from build123d import *

# Parameters (mm, degrees)
CROQUIS1_W              = 35
CROQUIS1_H              = 15
CROQUIS1_R              = 1.5
SALIENTE_EXTRUIR1_DEPTH = 4
CROQUIS2_W              = 4
CROQUIS2_H              = 15
SALIENTE_EXTRUIR2_DEPTH = 60
SALIENTE_EXTRUIR3_DEPTH = 15
CROQUIS4_R              = 2.85
CORTAR_EXTRUIR1_DEPTH   = 1.65
CROQUIS5_W              = 5
CROQUIS5_H              = 22
CORTAR_EXTRUIR2_DEPTH   = 22
CORTAR_EXTRUIR5_REACH   = 73.507
CROQUIS6_R              = 1.5
CROQUIS7_R              = 2.5
CORTAR_EXTRUIR6_DEPTH   = 2
CROQUIS9_W              = 13
CROQUIS9_H              = 14.4
SALIENTE_EXTRUIR4_DEPTH = 10


with BuildPart() as part:
    # Croquis1 → Saliente-Extruir1 (new body)
    with BuildSketch(Plane(origin=(0, 0, 0), x_dir=(1, 0, 0), z_dir=(0, 1, 0))):
        Rectangle(CROQUIS1_W, CROQUIS1_H)
        with Locations(Location((5.5, 3.75, 0), (0, 0, 270))):
            Circle(CROQUIS1_R, mode=Mode.SUBTRACT)
        with Locations(Location((13.5, 3.75, 0), (0, 0, 270))):
            Circle(CROQUIS1_R, mode=Mode.SUBTRACT)
    extrude(amount=SALIENTE_EXTRUIR1_DEPTH)

    # Croquis2 → Saliente-Extruir2 (add)
    with BuildSketch(Plane(origin=(0, 4, 0), x_dir=(1, 0, 0), z_dir=(0, 1, 0))):
        with Locations((-15.5, 0)):
            Rectangle(CROQUIS2_W, CROQUIS2_H)
    extrude(amount=SALIENTE_EXTRUIR2_DEPTH)

    # Croquis3 → Saliente-Extruir3 (add)
    with BuildSketch(Plane.XY.offset(7.5)):
        Polygon((-13.5, 4), (-13.5, 30), (1.5, 4), align=None)
    extrude(amount=-SALIENTE_EXTRUIR3_DEPTH)

    # Croquis4 → Cortar-Extruir1 (cut)
    with BuildSketch(Plane(origin=(0, 4, 0), x_dir=(1, 0, 0), z_dir=(0, 1, 0))):
        with Locations(Location((5.5, 3.75, 0), (0, 0, 270))):
            Circle(CROQUIS4_R)
        with Locations(Location((13.5, 3.75, 0), (0, 0, 270))):
            Circle(CROQUIS4_R)
    extrude(amount=-CORTAR_EXTRUIR1_DEPTH, mode=Mode.SUBTRACT)

    # Croquis5 → Cortar-Extruir2 (cut)
    with BuildSketch(Plane(origin=(17.5, 0, 0), x_dir=(0, 0, -1), z_dir=(1, 0, 0))):
        with Locations((-5, 11)):
            Rectangle(CROQUIS5_W, CROQUIS5_H)
    extrude(amount=-CORTAR_EXTRUIR2_DEPTH, mode=Mode.SUBTRACT)

    # Croquis6 → Cortar-Extruir5 (cut, up to next)
    with BuildSketch(Plane(origin=(-13.5, 0, 0), x_dir=(0, 0, -1), z_dir=(1, 0, 0)), mode=Mode.PRIVATE) as cortar_extruir5_sk1:
        with Locations((-3.3, 59.52)):
            Circle(CROQUIS6_R)
    cortar_extruir5_tool1 = extrude(cortar_extruir5_sk1.sketch, amount=-CORTAR_EXTRUIR5_REACH, mode=Mode.PRIVATE) & part.part
    # Croquis6 → Cortar-Extruir5 (cut, up to next)
    with BuildSketch(Plane(origin=(-13.5, 0, 0), x_dir=(0, 0, -1), z_dir=(1, 0, 0)), mode=Mode.PRIVATE) as cortar_extruir5_sk2:
        with Locations((3.3, 52.48)):
            Circle(CROQUIS6_R)
    cortar_extruir5_tool2 = extrude(cortar_extruir5_sk2.sketch, amount=-CORTAR_EXTRUIR5_REACH, mode=Mode.PRIVATE) & part.part
    add(cortar_extruir5_tool1.solids().sort_by_distance((-13.5, 59.52, 3.3))[0], mode=Mode.SUBTRACT)
    add(cortar_extruir5_tool2.solids().sort_by_distance((-13.5, 52.48, -3.3))[0], mode=Mode.SUBTRACT)

    # Croquis7 → Cortar-Extruir6 (cut)
    with BuildSketch(Plane.ZY.offset(17.5)):
        with Locations((-3.3, 52.48)):
            Circle(CROQUIS7_R)
        with Locations((3.3, 59.52)):
            Circle(CROQUIS7_R)
    extrude(amount=-CORTAR_EXTRUIR6_DEPTH, mode=Mode.SUBTRACT)

    # Croquis9 → Saliente-Extruir4 (add)
    with BuildSketch(Plane.XY.offset(7.5)):
        with Locations((-11, 7.2)):
            Rectangle(CROQUIS9_W, CROQUIS9_H)
    extrude(amount=SALIENTE_EXTRUIR4_DEPTH)


solid = part.part
Input: part model. Units: mm. Frame: model coordinates. A direction names the side the tool comes from. Give positions to 0.01 mm unless a question says otherwise; leave off trailing zeros. Write each loop counter-clockwise with the first axis right and the second up, starting at its lowest first coordinate (ties: lowest second). Pieces come first, ordered by that corner, then holes.
Q1. First-contact query: P1, Ø1, axis at y = 57.5, z = -1, coming from the +X side; P2, Ø3, axis at x = 8.5, z = -1.5, coming from the +Y side; P3, Ø11, axis at x = -14, z = 13.5, coming from the +Y side. Flat tips, straight axial feed; report the tip coordinate or a pass-through.
Q2. Set-up query: faces 4 (the face through (9, 4, -3)), 5 (the face through (-15.5, 51, -2)), 6 (the face through (4, 2, 2.5)), 7 (the face through (12, 2.35, -3)). Return all of +Z, -Z, +X, -X, +Y, -Y with unobstructed straight access to the full face (end or side cutting, diameter ignored); none if empty.
Q3. Material intervals for probe 1 along X at (y, z) = (3.05, -3.75); probe 2 along X at (y, z) = (1.15, -3.75); probe 3 along Y at (x, z) = (-16.3, 3.3), sorted ascending.
Q4. Pull-direction query (Y, two-part tool) for faces 1 (the face through (4, 2.35, -3)), 2 (the face through (-14.486, 61.007, 3.495)), 3 (the face through (-10, 18, -7.5)); classes: pulls with the +Y half, pulls with the -Y half, needs draft (parallel to the pull), parting line crosses it, or undercut.
Q5. Section A-A, the plane y = 52.48. Output: boundary loops of the cut face in (x, z), plus the area to 3 significant figures.
Q6. Section B-B, the plane z = 3.3. Output: boundary loops of the cut face in (x, y).
Q7. Section C-C, the plane x = 5.5. Output: boundary loops of the cut face in (y, z).
Q8. Section D-D, the plane z = -3.75. State how many separate pieces and enclosed holes the cut face has, plus the area to 3 significant figures.
Filled in:
1. P1: stops at x = -13.5
1. P2: stops at y = 4
1. P3: stops at y = 14.4
2. face 4: +Z, -Z, +X, +Y
2. face 5: -X
2. face 6: +Z, +X, +Y, -Y
2. face 7: +Y
3. probe 1: x = -17.5 to 2.65, 8.35 to 10.65, 16.35 to 17.5
3. probe 2: x = -17.5 to 4, 7 to 12, 15 to 17.5
3. probe 3: y = 0 to 57.02, 62.02 to 64
4. face 1: pulls with the +Y half
4. face 2: undercut
4. face 3: needs draft
5. outline: (-17.5, -7.5) - (-13.5, -7.5) - (-13.5, -4.8) - (-15.5, -4.8) - (-15.5, -5.8) - (-17.5, -5.8) - close; (-17.5, -0.8) - (-15.5, -0.8) - (-15.5, -1.8) - (-13.5, -1.8) - (-13.5, 7.5) - (-17.5, 7.5) - close
5. area: 44.0 mm2
6. outline: (-17.5, 0) - (-4.5, 0) - (-4.5, 14.4) - (-13.5, 30) - (-13.5, 58.02) - (-15.5, 58.02) - (-15.5, 57.02) - (-17.5, 57.02) - close; (-17.5, 62.02) - (-15.5, 62.02) - (-15.5, 61.02) - (-13.5, 61.02) - (-13.5, 64) - (-17.5, 64) - close
7. outline: (0, -7.5) - (4, -7.5) - (4, -6.6) - (2.35, -6.6) - (2.35, -5.25) - (0, -5.25) - close; (0, -2.25) - (2.35, -2.25) - (2.35, -0.9) - (4, -0.9) - (4, 2.5) - (0, 2.5) - close
8. separate pieces: 4
8. enclosed holes: 0
8. area: 527 mm2
